from build123d import *

# Parameters (mm, degrees)
F0_W        = 108.7058566231
F0_H        = 36.235285541
F1_DEPTH    = 304.8
F3_DEPTH    = 304.8
F4_T1_DEPTH = 31.2448363711
F4_T3_DEPTH = 315.5177056065
F6_D        = 12.7


# Not quite as in the source:
# - a fillet or chamfer that OpenCascade refuses, or shapes differently, is made with other operations: its cross-section is extruded or revolved along the edge and cut away or added
# - a feature names something its author has since deleted; it is built from what else it names


with BuildPart() as f1:
    # F0 (on Front) → F1 (new body)
    with BuildSketch(Plane.XZ):
        with Locations((54.3529283115, 18.1176427705)):
            Rectangle(F0_W, F0_H)
    extrude(amount=-F1_DEPTH)

    # F2 (on face) → F3 (join)
    with BuildSketch(Plane.XZ):
        Polygon((210.6682882407, -76.6480192542), (108.3266659877, 36.8101285866), (108.3266659877, 36.235285541), (108.7058566231, 36.235285541), (108.7058566231, 25.7386137456), (210.6682882407, -81.7645564675), align=None)
    extrude(amount=-F3_DEPTH)

    # F4: chamfer of 5.08 on 3 edges, made by hand

    # F4_s2 → F4_t1 (cut)
    with BuildSketch(Plane.XY.offset(-94.8287060464)):
        Polygon((205.5882882407, 0), (210.6682882407, 5.08), (210.6682882407, 0), align=None)
        Polygon((205.5882882407, 304.8), (210.6682882407, 299.72), (210.6682882407, 304.8), align=None)
    extrude(amount=F4_T1_DEPTH, mode=Mode.SUBTRACT)

    # F4_s4 → F4_t3 (cut)
    with BuildSketch(Plane.XZ.offset(-310.1588528033)):
        Polygon((209.3604296259, -75.1980987546), (210.6682882407, -78.6006491759), (210.6682882407, -76.6480192542), align=None)
    extrude(amount=F4_T3_DEPTH, mode=Mode.SUBTRACT)

    # F6 (through all)
    with Locations(Plane.XY.offset(36.235285541)):
        with Locations((54.1633329939, 228.6), (54.1633329939, 152.4), (54.1633329939, 279.4), (54.1633329939, 254), (54.1633329939, 177.8), (54.1633329939, 203.1635642052), (54.1633329939, 127.0884871483), (54.1633329939, 101.6), (54.1633329939, 50.8), (54.1633329939, 25.4), (54.1633329939, 76.2)):
            Hole(F6_D / 2)


solid = f1.part
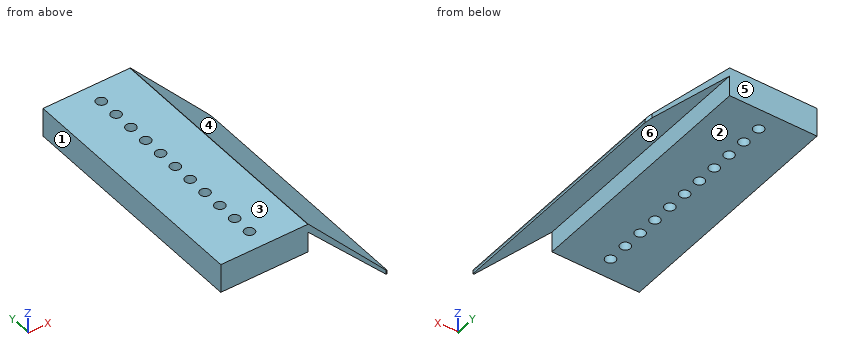
Work out the finished part from the listing and answer in its coordinate system (mm). Face numbers are marked on the shaded views. A direction names the side the tool comes from. Round coordinates to 2 decimals unless told otherwise and drop trailing zeros. Write each loop counter-clockwise with the first axis right and the second up, starting at its lowest first coordinate (ties: lowest second). Pieces come first, ordered by that corner, then holes.
1) Given pin 1 Ø20.5 at (x, y) = (54.16, 101.6) entering from +Z; pin 2 Ø16.5 at (x, y) = (54.16, 25.4) entering from -Z; pin 3 Ø20.5 at (y, z) = (142.5, 10) entering from +X; pin 4 Ø7.5 at (x, y) = (54.16, 127.09) entering from +Z, each flat-ended and moving along its own axis, determine where each tip first touches the part or whether it passes through.
2) A cutting plane is placed at C-C (x = 99). Give the vertices of the cut face in (y, z).
3) A cutting plane is placed at D-D (z = -47). Give the vertices of the cut face in (x, y).
4) A cutting plane is placed at A-A (y = 228.6). Give the vertices of the cut face in (x, z).
5) The mould has two halves that part along X. Classify the marked faces 4, 5 and 6: pulls with the +X half, pulls with the -X half, needs draft (parallel to the pull), parting line crosses it, or undercut.
6) A cutting plane is placed at B-B (y = 114). Give the vertices of the cut face in (x, z).
7) Straight lines are drawn through the part: line 1 (X direction, y = 279.4, z = 9); line 2 (X direction, y = 81.5, z = 25.5); line 3 (Z direction, x = 29, y = 215). For each, find the intervals that lie inside material, in ascending order.
8) A tool of negligible diameter and unlimited length cuts with its end or side. For the marked faces 1, 2 and 3, from which of +Z, -Z, +X, -X, +Y, -Y can it reach the whole face along a straight path? Write none if from no direction.
Completed:
1. pin 1: stops at z = 36.24
1. pin 2: stops at z = 0
1. pin 3: stops at x = 141.76
1. pin 4: passes through
2. outline: (0, 0) - (304.8, 0) - (304.8, 36.24) - (0, 36.24) - close
3. outline: (177.7, 0) - (183.93, 0) - (183.93, 304.8) - (177.7, 304.8) - close
4. outline: (0, 0) - (47.81, 0) - (47.81, 36.24) - (0, 36.24) - close; (60.51, 0) - (108.71, 0) - (108.71, 25.74) - (210.67, -81.76) - (210.67, -78.6) - (209.36, -75.2) - (108.33, 36.81) - (108.33, 36.24) - (60.51, 36.24) - close
5. face 4: pulls with the +X half
5. face 5: needs draft
5. face 6: undercut
6. outline: (0, 0) - (108.71, 0) - (108.71, 25.74) - (210.67, -81.76) - (210.67, -78.6) - (209.36, -75.2) - (108.33, 36.81) - (108.33, 36.24) - (0, 36.24) - close
7. line 1: x = 0 to 47.81, 60.51 to 108.71, 124.58 to 133.41
7. line 2: x = 0 to 50.67, 57.66 to 108.71, 108.93 to 118.53
7. line 3: z = 0 to 36.24
8. face 1: +Z, -Z, -X, +Y, -Y
8. face 2: -Z, -X, +Y, -Y
8. face 3: +Z, -X, +Y, -Y
